```python
from build123d import *

# Parameters (mm, degrees)
CONTINUOUS_OUTER_IMPACT_SKIN_DEPTH = 282


with BuildPart() as part:
    # Continuous outer impact skin profile → Continuous outer impact skin (new body)
    with BuildSketch(Plane.XY):
        with BuildLine():
            Line((152, 3), (140.245569122, 3))
            ThreePointArc((140.245569122, 3), (140.001830435, 3.014907697), (139.761725331, 3.059408547))
            Line((139.761725331, 3.059408547), (121.342178632, 7.651917339))
            ThreePointArc((121.342178632, 7.651917339), (121.012549136, 7.765417876), (120.707636616, 7.934433647))
            Line((120.707636616, 7.934433647), (105.352434752, 18.291648082))
            ThreePointArc((105.352434752, 18.291648082), (105.032140958, 18.560406486), (104.774724366, 18.889884698))
            Line((104.774724366, 18.889884698), (94, 36.133048143))
            Line((94, 36.133048143), (93.151951903, 35.603128878))
            Line((93.151951903, 35.603128878), (103.926676269, 18.359965433))
            ThreePointArc((103.926676269, 18.359965433), (104.312801157, 17.865748115), (104.793241848, 17.462610509))
            Line((104.793241848, 17.462610509), (120.148443712, 7.105396074))
            ThreePointArc((120.148443712, 7.105396074), (120.605812493, 6.851872418), (121.100256736, 6.681621612))
            Line((121.100256736, 6.681621612), (139.519803435, 2.08911282))
            ThreePointArc((139.519803435, 2.08911282), (139.879961091, 2.022361545), (140.245569122, 1.999999999))
            Line((140.245569122, 1.999999999), (152, 1.999999999))
            Line((152, 1.999999999), (152, 3))
        make_face()
    extrude(amount=CONTINUOUS_OUTER_IMPACT_SKIN_DEPTH)


solid = part.part
```
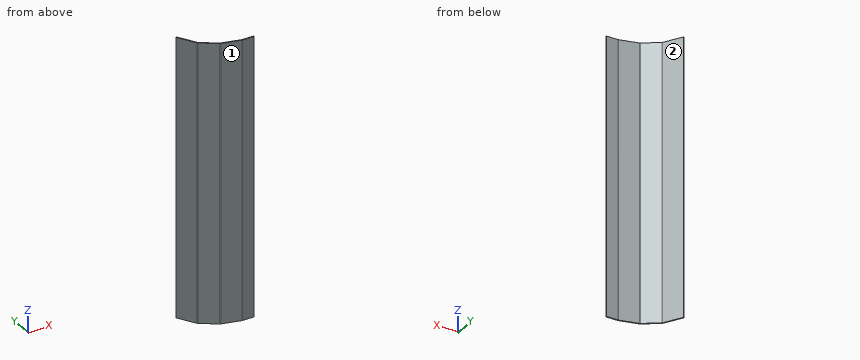
Model file for the job. Use its own axes, mm. Face numbers are marked on the shaded views. Round coordinates to 2 decimals unless told otherwise and drop trailing zeros. Write each loop counter-clockwise with the first axis right and the second up, starting at its lowest first coordinate (ties: lowest second). Pieces come first, ordered by that corner, then holes. Notation, with made-up numbers: M 60.5,-20.75 L 79.5,-20.75 A21 cw 79.5,1.25 Z; hole C 75.25,87 d9. An arc over 180 degrees is marked long. Put each result on its own line as item: value.
Item 1: Probe L1, parallel to Y at x = 111, z = 213; L2, parallel to X at y = 29.5, z = 12; L3, parallel to X at y = 27, z = 135.5. List the from-to ranges inside material, lowest first. Write a range as from..to.
Responses:
L1: 13.28..14.48
L2: 96.97..98.14
L3: 98.53..99.71
Item 2: Mould opens along Y. For the marked faces 1 and 2 say: +Y half, -Y half, draft (parallel to the pull), parting line (faces both ways), or undercut.
Responses:
face 1: -Y half
face 2: +Y half
Item 3: Cut at B-B (x = 135.5). List the corners of the cut face in (y, z), and give its area (3 significant figures).
Responses:
outline: M 3.09,0 L 4.12,0 L 4.12,282 L 3.09,282 Z
area: 291 mm²
Item 4: Flat gauge pins, fed straight in: P1, Ø1, axis at y = 29.5, z = 102.5, coming from the +X side; P2, Ø1.5, axis at y = 32.5, z = 221.5, coming from the +X side; P3, Ø1.5, axis at x = 133.5, z = 212, coming from the +Y side. Where does each tip first touch, or does it go through?
Responses:
P1: x = 98.46
P2: x = 96.74
P3: y = 4.81
Item 5: Cut at C-C (y = 27). List the corners of the cut face in (x, z).
Responses:
outline: M 98.53,0 L 99.71,0 L 99.71,282 L 98.53,282 Z
Item 6: Cut at A-A (z = 84). List the corners of the cut face in (x, y), and give its area (3 significant figures).
Responses:
outline: M 93.15,35.6 L 103.93,18.36 A3 ccw 104.79,17.46 L 120.15,7.11 A3 ccw 121.1,6.68 L 139.52,2.09 A3 ccw 140.25,2 L 152,2 L 152,3 L 140.25,3 A2 cw 139.76,3.06 L 121.34,7.65 A2 cw 120.71,7.93 L 105.35,18.29 A2 cw 104.77,18.89 L 94,36.13 Z
area: 72.1 mm²
